```python
from build123d import *

# Parameters (mm, degrees)
SKETCH_1_W          = 23.45
SKETCH_1_H          = 10
EXTRUDE_1_DEPTH     = 58
EXTRUDE_2_DEPTH     = 58
SKETCH_5_W          = 23.35
SKETCH_5_H          = 55
CUT_EXTRUDE_2_DEPTH = 9.01


with BuildPart() as part:
    # 草圖1 → 填料-伸長1 (new body)
    with BuildSketch(Plane(origin=(0, 0, 0), x_dir=(1, 0, 0), z_dir=(0, 1, 0))):
        Rectangle(SKETCH_1_W, SKETCH_1_H)
    extrude(amount=EXTRUDE_1_DEPTH)

    # 草圖3 → 填料-伸長2 (add)
    with BuildSketch(Plane(origin=(0, 58, 0), x_dir=(1, 0, 0), z_dir=(0, 1, 0))):
        Polygon((-11.725, 0.4), (-12.725, 0.4), (-12.725, 1.4), (-13.725, 1.4), (-13.725, -1.60013631), (-12.725, -1.60013631), (-12.725, -0.6), (-11.725, -0.6), align=None)
    extrude(amount=-EXTRUDE_2_DEPTH)

    # 草圖5 → 除料-伸長2 (cut)
    with BuildSketch(Plane(origin=(0, 0, -5), x_dir=(-1, 0, 0), z_dir=(0, 0, -1))):
        with Locations((-0.05, 27.5)):
            Rectangle(SKETCH_5_W, SKETCH_5_H)
    extrude(amount=-CUT_EXTRUDE_2_DEPTH, mode=Mode.SUBTRACT)


solid = part.part
```
Here's how the part is built. I have some questions about the finished solid (model axes, mm). A direction names the side the tool comes from. Coordinates: 2 decimals unless noted, no trailing zeros. Order: outer loops, then holes, each group sorted by start corner. A loop starts at its lowest first (then second) coordinate and runs counter-clockwise, first axis right, second up.
Item 1: I'm going to push flat-ended pins straight in: pin 1 Ø1 at (y, z) = (26, 3) entering from -X (3 decimals); pin 2 Ø1.1 at (x, y) = (-13, 33) entering from -Z; pin 3 Ø3 at (y, z) = (32.5, -0.5) entering from +X (3 decimals). Where does each tip first touch, or does it pass through?
Response values:
pin 1: stops at x = -11.725
pin 2: stops at z = -1.4
pin 3: stops at x = -11.625
Item 2: If we section it at A-A, the plane y = 14: List the corners of the cut face in (x, z) for me (3 decimals).
Response values:
outline: (-13.725, -1.4) - (-12.725, -1.4) - (-12.725, -0.4) - (-11.725, -0.4) - (-11.725, -5) - (-11.625, -5) - (-11.625, 4.01) - (11.725, 4.01) - (11.725, 5) - (-11.725, 5) - (-11.725, 0.6) - (-12.725, 0.6) - (-12.725, 1.6) - (-13.725, 1.6) - close
Item 3: If we section it at C-C, the plane z = -3.25: List the corners of the cut face in (x, y) for me (3 decimals).
Response values:
outline: (-11.725, 0) - (-11.625, 0) - (-11.625, 55) - (11.725, 55) - (11.725, 58) - (-11.725, 58) - close
Item 4: I need wall thicknesses on probe 1 along Y at (x, z) = (-0.5, -3.75); probe 2 along Z at (x, y) = (10.5, 12.5); probe 3 along X at (y, z) = (41.5, 0.5) (3 decimals). Which ranges of each line are inside material? Lowest first, please.
Response values:
probe 1: y = 55 to 58
probe 2: z = 4.01 to 5
probe 3: x = -13.725 to -11.625
Item 5: Which directions (+Z, -Z, +X, -X, +Y, -Y) give clear straight access to the entire face, cutting with the end or side of a thin tool? Please do faces 1 (the face through (-12.725, 29, -1)), 2 (the face through (-11.625, 27, 0)), 3 (the face through (-13, 29, -1.4)).
Response values:
face 1: -Z, +Y, -Y
face 2: -Z, +X, -Y
face 3: -Z, -X, +Y, -Y
Item 6: If we section it at B-B, the plane x = 1.5: List the corners of the cut face in (y, z) for me.
Response values:
outline: (0, 4.01) - (55, 4.01) - (55, -5) - (58, -5) - (58, 5) - (0, 5) - close
